The model under review builds one solid part; all positions refer to its coordinate system, in mm. Coordinates: 2 decimals unless noted, no trailing zeros. Loops run counter-clockwise (first coordinate to the right, second up) from the corner with the lowest first, then second, coordinate; pieces in that order, holes last. Notation, with made-up numbers: (-10, 85) - (11, 85) arc R12 ccw to (11, 100) - close; hole circle Ø9 at (57, 89.5). An arc over 180 degrees is marked (long way). One line per item, written item: value. Start each with the question number.
1. We need section B-B, the plane x = 13.25. Give the boundary of the cut face in (y, z).
2. Mouldability with a two-part tool opening along Z and no side actions: class faces 1 (the face through (8, 0.794, 106)), 2 (the face through (4.4, 0.3, 215.9)), 3 (the face through (7.963, 0.402, 211.224)) as +Z half, -Z half, draft (parallel to the pull), parting line (faces both ways), or undercut.
3. Insertion check: P1, Ø4, axis at y = 6.5, z = 139.5, coming from the +X side; P2, Ø3, axis at x = 13.5, z = 137.5, coming from the -Y side. Each pin has a flat end and moves straight along its axis. Give the tip position at first contact, or say it passes through.
4. We need section A-A, the plane z = 198. Give the boundary of the cut face in (x, y) (3 decimals).
5. To check wall thickness, follow line 1 (Y direction, x = 0.45, z = 203.2) (3 decimals); line 2 (X direction, y = 4, z = 96). State the ranges of each line that lie inside material, in increasing order.
Autodesk Inventor part; units mm, degrees
ref_plane "YZ Plane" through (0, 0, 0) normal (1, 0, 0) x (0, 1, 0)
ref_plane "XZ Plane" through (0, 0, 0) normal (0, 1, 0) x (-1, 0, 0)
ref_plane "XY Plane" through (0, 0, 0) normal (0, 0, 1) x (1, 0, 0)
sketch "Sketch1" plane through (0, 0, 0) normal (0, 0, 1) x (1, 0, 0)
  line L0 (0, 0) -> (0, 15.875)
  line L1 (0, 15.875) -> (0.7937, 15.875)
  line L2 (0.7937, 15.875) -> (0.7938, 0.7937)
  line L3 (0.7938, 0.7937) -> (15.875, 0.7937)
  line L4 (15.875, 0.7937) -> (15.875, 0)
  line L5 (15.875, 0) -> (0, 0)
  dimension "d0" = 15.875
  dimension "d1" = 0.7937
extrude "Extrusion1" add sketch "Sketch1" along normal blind 215.9
sketch "Sketch2" plane through (0.7938, 0.7937, 0) normal (0, 1, 0) x (1, 0, 0)
  line L0 (0, 0) -> (15.0812, 0)
  line L1 (15.0812, -215.9) -> (0, -215.9)
  line L2 (7.5406, 0) -> (7.5406, -215.9) construction
  circle A0 centre (7.5406, -25.4) radius 1.7145
  circle A1 centre (7.5406, -209.55) radius 1.7145
  point P0 (-0.7938, 0)
  dimension "d4" = 25.4
  dimension "d5" = 3.429
  dimension "d6" = 215.9
  dimension "d28" = 6.35
sketch "Sketch3" plane through (0.7938, 0.7937, 0) normal (1, 0, 0) x (0, 0, -1)
  line L0 (0, 15.0812) -> (0, 0)
  line L1 (-215.9, 0) -> (-215.9, 15.0812)
  line L2 (-215.9, 7.5406) -> (0, 7.5406) construction
  circle A0 centre (-25.4, 7.5406) radius 1.7145
  circle A1 centre (-114.3, 7.5406) radius 1.7145
  circle A2 centre (-203.2, 7.5406) radius 1.7145
  point P0 (0, -0.7937)
  dimension "d14" = 3.429
  dimension "d15" = 25.4
  dimension "d16" = 215.9
  dimension "d19" = 88.9
extrude "Extrusion2" cut sketch "Sketch2" against normal through all
extrude "Extrusion3" cut sketch "Sketch3" against normal through all
properties part number "Hopper Bracing Right Leg P13" material "Aluminum 6061"
Findings below:
1. outline: (0, 0) - (0.79, 0) - (0.79, 215.9) - (0, 215.9) - close
2. face 1: draft
2. face 2: +Z half
2. face 3: undercut
3. P1: x = 0.79
3. P2: y = 0
4. outline: (0, 0) - (15.875, 0) - (15.875, 0.794) - (0.794, 0.794) - (0.794, 15.875) - (0, 15.875) - close
5. line 1: 0 to 6.62, 10.049 to 15.875
5. line 2: 0 to 0.79
